from build123d import *

# Parameters (mm, degrees)
SKETCH1_W           = 45
SKETCH1_H           = 8
BOSS_EXTRUDE1_DEPTH = 1.5
SKETCH2_W           = 3
SKETCH2_H           = 8
BOSS_EXTRUDE2_DEPTH = 14
SKETCH3_W           = 8
SKETCH3_H           = 2
BOSS_EXTRUDE3_DEPTH = 13


with BuildPart() as part:
    # Sketch1 → Boss-Extrude1 (new body)
    with BuildSketch(Plane(origin=(0, 0, 0), x_dir=(1, 0, 0), z_dir=(0, 1, 0))):
        Rectangle(SKETCH1_W, SKETCH1_H)
    extrude(amount=BOSS_EXTRUDE1_DEPTH)

    # Sketch2 → Boss-Extrude2 (add)
    with BuildSketch(Plane(origin=(0, 1.5, 0), x_dir=(1, 0, 0), z_dir=(0, 1, 0))):
        with Locations((21, 0)):
            Rectangle(SKETCH2_W, SKETCH2_H)
    extrude(amount=BOSS_EXTRUDE2_DEPTH)

    # Sketch3 → Boss-Extrude3 (add)
    with BuildSketch(Plane.ZY.offset(-19.5)):
        with Locations((0, 14.5)):
            Rectangle(SKETCH3_W, SKETCH3_H)
    extrude(amount=BOSS_EXTRUDE3_DEPTH)


solid = part.part
Read the model definition and answer for the solid it produces. Units are mm, in the model's axes. A direction names the side the tool comes from. Coordinates: 2 decimals unless noted, no trailing zeros. Write each loop counter-clockwise with the first axis right and the second up, starting at its lowest first coordinate (ties: lowest second). Pieces come first, ordered by that corner, then holes. Notation, with made-up numbers: M -32,-20.75 L -26,-20.75 A34 cw -26,13.25 Z; hole C 22,14 d2. An arc over 180 degrees is marked long. Use a Markdown table: item, result.
Q1. Each of these flat-tipped pins is pushed along its axis until it touches: pin 1 Ø1.5 at (x, z) = (-8, -0.5) entering from +Y; pin 2 Ø1.6 at (y, z) = (15, 1) entering from -X. Where does it stop, or does it pass through?
Answer block:
| item | result |
|---|---|
| pin 1 | stops at y = 1.5 |
| pin 2 | stops at x = 6.5 |
Q2. The part is cut by section D-D, the plane x = -12.5. Write down the section's boundary in (y, z), then the cut area to 3 significant figures.
Answer block:
| item | result |
|---|---|
| outline | M 0,-4 L 1.5,-4 L 1.5,4 L 0,4 Z |
| area | 12.0 mm2 |
Q3. The part is cut by section C-C, the plane y = 11. Write down the section's boundary in (x, z), then the cut area to 3 significant figures.
Answer block:
| item | result |
|---|---|
| outline | M 19.5,-4 L 22.5,-4 L 22.5,4 L 19.5,4 Z |
| area | 24.0 mm2 |
Q4. The part is cut by section B-B, the plane z = 0.5. Write down the section's boundary in (x, y), then the cut area to 4 significant figures.
Answer block:
| item | result |
|---|---|
| outline | M -22.5,0 L 22.5,0 L 22.5,15.5 L 6.5,15.5 L 6.5,13.5 L 19.5,13.5 L 19.5,1.5 L -22.5,1.5 Z |
| area | 135.5 mm2 |
Q5. Straight lines are drawn through the part: L1, parallel to Y at x = 8.5, z = -1.5; L2, parallel to X at y = 14, z = 3; L3, parallel to Y at x = -21, z = 3.5. For each, find the intervals that lie inside material, in ascending order. Write a range as [from, to].
Answer block:
| item | result |
|---|---|
| L1 | y = [0, 1.5], [13.5, 15.5] |
| L2 | x = [6.5, 22.5] |
| L3 | y = [0, 1.5] |
Q6. Determine the mould class of faces 1 (the face through (-22.5, 1, 0)), 2 (the face through (13, 13.5, 0)), 3 (the face through (15, 15.5, 0)) for opening direction Y: released by +Y, released by -Y, zero draft, split by the parting line, or undercut.
Answer block:
| item | result |
|---|---|
| face 1 | zero draft |
| face 2 | undercut |
| face 3 | released by +Y |
Q7. The part is cut by section A-A, the plane x = 17.5. Write down the section's boundary in (y, z).
Answer block:
| item | result |
|---|---|
| outline | M 0,-4 L 1.5,-4 L 1.5,4 L 0,4 Z; M 13.5,-4 L 15.5,-4 L 15.5,4 L 13.5,4 Z |
Q8. Which of the six approach directions +Z, -Z, +X, -X, +Y, -Y give full straight-line access (tool end or side, diameter ignored) to faces 4 (the face through (-2, 1.5, 0)), 5 (the face through (6.5, 15, 0)), 6 (the face through (22.5, 8, 0))?
Answer block:
| item | result |
|---|---|
| face 4 | +Z, -Z, -X |
| face 5 | +Z, -Z, -X, +Y |
| face 6 | +Z, -Z, +X, +Y, -Y |
